from build123d import *


with BuildPart() as part:
    # Sketch1 → Revolve1 (revolve)
    with BuildSketch(Plane(origin=(0, 0, 0), x_dir=(0, 0, -1), z_dir=(1, 0, 0))):
        Polygon((-4, 0), (-4, 2), (81.5, 2), (81.5, 5), (84, 5), (84, 0), align=None)
    revolve(axis=Axis((0, 0, -84), (0, 0, 1)))

    # Sketch2 → Revolve2 (revolve)
    with BuildSketch(Plane(origin=(0, 0, 0), x_dir=(0, 0, -1), z_dir=(1, 0, 0))):
        with BuildLine():
            Line((-16, 0), (-16, 1.5705))
            Line((-16, 1.5705), (-15.5705, 2))
            Line((-15.5705, 2), (-6.298990968, 2))
            Line((-6.298990968, 2), (-5.266277265, 1.624122952))
            ThreePointArc((-5.266277265, 1.624122952), (-5.198928479, 1.606076899), (-5.129469208, 1.6))
            Line((-5.129469208, 1.6), (-4.4, 1.6))
            ThreePointArc((-4.4, 1.6), (-4.117157288, 1.717157288), (-4, 2))
            Line((-4, 2), (-3, 2))
            Line((-3, 2), (-3, 0))
            Line((-3, 0), (-16, 0))
        make_face()
    revolve(axis=Axis((0, 0, 3), (0, 0, 1)))


solid = part.part
Geometry check sheet. Reference: the model listing, model coordinates, mm. Give positions to 0.01 mm unless a question says otherwise; leave off trailing zeros. Loops run counter-clockwise (first coordinate to the right, second up) from the corner with the lowest first, then second, coordinate; pieces in that order, holes last.
(1) Release check for a two-part mould opening along Z. For faces 1 (the cylindrical face through (4.88, -1.08, -82.77)), 2 (the cylindrical face through (0.97, -1.27, 4.76)), 3 (the flat face through (0, 0, 16)), 4 (the flat face through (0, 0, -84)) record: released by +Z, released by -Z, zero draft, split by the parting line, or undercut.
From the geometry:
face 1: zero draft
face 2: undercut
face 3: released by +Z
face 4: released by -Z
(2) Thickness scan on L1, parallel to Y at x = -1.25, z = -26; L2, parallel to Z at x = -2, y = 2.5; L3, parallel to X at y = 0.75, z = -18.5. Record the ranges inside material, lowest first.
From the geometry:
L1: y = -1.56 to 1.56
L2: z = -84 to -81.5
L3: x = -1.85 to 1.85
(3) Section check C-C on z = -38. Record the cut outline in (x, y), then the cut area to 3 significant figures.
From the geometry:
outline: circle Ø4 at (0, 0)
area: 12.6 mm2
(4) Section check A-A on y = 0. Record the cut outline in (x, z), then the cut area to 3 significant figures.
From the geometry:
outline: (-5, -84) - (5, -84) - (5, -81.5) - (2, -81.5) - (2, 4) arc R0.4 cw to (1.6, 4.4) - (1.6, 5.13) arc R0.4 cw to (1.62, 5.27) - (2, 6.3) - (2, 15.57) - (1.57, 16) - (-1.57, 16) - (-2, 15.57) - (-2, 6.3) - (-1.62, 5.27) arc R0.4 cw to (-1.6, 5.13) - (-1.6, 4.4) arc R0.4 cw to (-2, 4) - (-2, -81.5) - (-5, -81.5) - close
area: 413 mm2
(5) Depth check by flat-ended pin: pin 1 Ø1 at (x, z) = (2, -30) entering from +Y; pin 2 Ø4 at (x, z) = (0, -38) entering from +Y; pin 3 Ø6 at (y, z) = (3.5, -65) entering from -X. Enter the tip coordinate at first touch or a pass-through.
From the geometry:
pin 1: stops at y = 1.32
pin 2: stops at y = 2
pin 3: stops at x = -1.94
